```python
from build123d import *

# Parameters (mm, degrees)
RESSALTO_EXTRUS_O1_DEPTH = 52
ESBO_O2_R                = 2
CORTE_EXTRUS_O1_DEPTH    = 100
ESBO_O3_W                = 41
ESBO_O3_H                = 32.35
CORTE_EXTRUS_O2_DEPTH    = 8.5
ESBO_O8_W                = 65
ESBO_O8_H                = 5.3
CORTE_EXTRUS_O6_DEPTH    = 39
ESBO_O9_W                = 0.75
ESBO_O9_H                = 56.4
CORTE_EXTRUS_O7_DEPTH    = 45
FILETE6_R                = 8


with BuildPart() as part:
    # Esboço1 → Ressalto-extrusão1 (new body)
    with BuildSketch(Plane(origin=(0, 0, 0), x_dir=(1, 0, 0), z_dir=(0, 1, 0))):
        Polygon((-32.5, -28.2), (-20.5, -28.2), (-20.5, 28.2), (-32.5, 28.2), (-32.5, 33.5), (32.5, 33.5), (32.5, 28.2), (20.5, 28.2), (20.5, -28.2), (32.5, -28.2), (32.5, -33.5), (-32.5, -33.5), align=None)
    extrude(amount=RESSALTO_EXTRUS_O1_DEPTH)

    # Esboço2 → Corte-extrusão1 (cut)
    with BuildSketch(Plane.XY.offset(33.5)):
        with Locations((27.8, 5.4)):
            Circle(ESBO_O2_R)
        with Locations((-27.8, 5.4)):
            Circle(ESBO_O2_R)
    extrude(amount=-CORTE_EXTRUS_O1_DEPTH, mode=Mode.SUBTRACT)

    # Esboço3 → Corte-extrusão2 (cut)
    with BuildSketch(Plane(origin=(0, 52, 0), x_dir=(1, 0, 0), z_dir=(0, 1, 0))):
        with Locations((0, -12.025)):
            Rectangle(ESBO_O3_W, ESBO_O3_H)
    extrude(amount=-CORTE_EXTRUS_O2_DEPTH, mode=Mode.SUBTRACT)

    # Esboço8 → Corte-extrusão6 (cut)
    with BuildSketch(Plane(origin=(0, 52, 0), x_dir=(1, 0, 0), z_dir=(0, 1, 0))):
        with Locations((0, -30.85)):
            Rectangle(ESBO_O8_W, ESBO_O8_H)
    extrude(amount=-CORTE_EXTRUS_O6_DEPTH, mode=Mode.SUBTRACT)

    # Esboço9 → Corte-extrusão7 (cut)
    with BuildSketch(Plane(origin=(0, 52, 0), x_dir=(1, 0, 0), z_dir=(0, 1, 0))):
        with Locations((-20.125, 0)):
            Rectangle(ESBO_O9_W, ESBO_O9_H)
        with Locations((20.125, 0)):
            Rectangle(ESBO_O9_W, ESBO_O9_H)
    extrude(amount=-CORTE_EXTRUS_O7_DEPTH, mode=Mode.SUBTRACT)

    # Filete6
    filete6_edges = [part.edges().sort_by_distance(p)[0] for p in [
        (19.75, 43.5, 12.025),
        (-19.75, 43.5, 12.025),
    ]]
    fillet(filete6_edges, radius=FILETE6_R)


solid = part.part
```
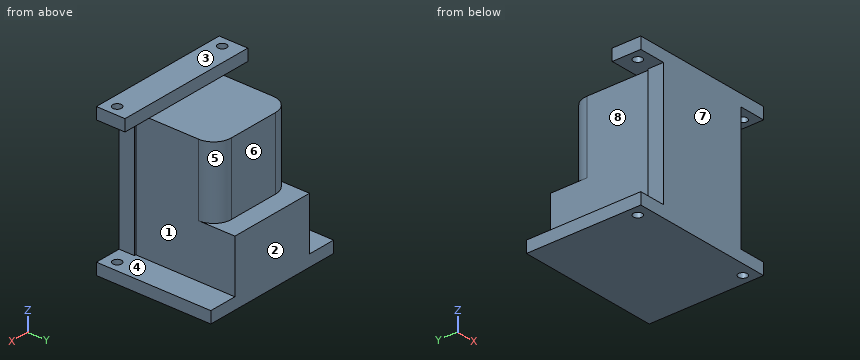
The listing builds one solid part. Answer for the finished solid, in the listing's coordinates (mm). Face numbers are marked on the shaded views. A direction names the side the tool comes from. Coordinates: 2 decimals unless noted, no trailing zeros. Loops run counter-clockwise (first coordinate to the right, second up) from the corner with the lowest first, then second, coordinate; pieces in that order, holes last. Notation, with made-up numbers: (9.25, 84.5) - (24.25, 84.5) arc R18 ccw to (24.25, 104.5) - close; hole circle Ø7 at (-18.5, 14.5). An arc over 180 degrees is marked (long way). Use a Markdown table: item, result. Add a question column.
1) The part is cut by section B-B, the plane y = 5.4. Give the vertices of the cut face in (x, z).
2) The part is cut by section C-C, the plane x = 27.8. Give the vertices of the cut face in (y, z).
3) The part is cut by section A-A, the plane z = -10. Give the vertices of the cut face in (x, y), and give its area (3 significant figures).
4) The mould has two halves that part along Z. Classify the marked faces 1, 2, 3 and 4: released by +Z, released by -Z, zero draft, split by the parting line, or undercut.
5) Find the intervals of material crossed by line 1 (Y direction, x = 27.8, z = -31.4); line 2 (X direction, y = 5, z = -29); line 3 (Z direction, x = 24, y = 10), in increasing order.
6) The part is cut by section D-D, the plane y = 22. Give the vertices of the cut face in (x, z).
7) Given pin 1 (3.5 mm diameter, centred on y = 3, z = 12.5, fed in from -X); pin 2 (5 mm diameter, centred on x = -6.5, y = 43, fed in from +Z); pin 3 (10 mm diameter, centred on y = 27.5, z = 22, fed in from +X), each flat-ended and moving along its own axis, determine where each tip first touches the part or whether it passes through.
8) For the marked faces 5, 6, 7 and 8, determine the directions among +Z, -Z, +X, -X, +Y, -Y from which every point of the face is accessible in a straight line to the end or side of a thin tool.
Here are the results:
| question | item | result |
|---|---|---|
| 1 | outline | (-32.5, -33.5) - (-29.8, -33.5) - (-29.8, -28.2) - (-32.5, -28.2) - close; (-32.5, 28.2) - (-29.8, 28.2) - (-29.8, 33.5) - (-32.5, 33.5) - close; (-25.8, -33.5) - (25.8, -33.5) - (25.8, -28.2) - (20.5, -28.2) - (20.5, 28.2) - (25.8, 28.2) - (25.8, 33.5) - (-25.8, 33.5) - (-25.8, 28.2) - (-20.5, 28.2) - (-20.5, -28.2) - (-25.8, -28.2) - close; (29.8, -33.5) - (32.5, -33.5) - (32.5, -28.2) - (29.8, -28.2) - close; (29.8, 28.2) - (32.5, 28.2) - (32.5, 33.5) - (29.8, 33.5) - close |
| 2 | outline | (0, -33.5) - (3.4, -33.5) - (3.4, -28.2) - (0, -28.2) - close; (0, 28.2) - (3.4, 28.2) - (3.4, 33.5) - (0, 33.5) - close; (7.4, -33.5) - (52, -33.5) - (52, -28.2) - (7.4, -28.2) - close; (7.4, 28.2) - (13, 28.2) - (13, 33.5) - (7.4, 33.5) - close |
| 3 | outline | (-20.5, 0) - (20.5, 0) - (20.5, 7) - (19.75, 7) - (19.75, 52) - (-19.75, 52) - (-19.75, 7) - (-20.5, 7) - close |
| 3 | area | 2,060 mm^2 |
| 4 | face 1 | undercut |
| 4 | face 2 | zero draft |
| 4 | face 3 | released by +Z |
| 4 | face 4 | undercut |
| 5 | line 1 | y = 0 to 3.4, 7.4 to 52 |
| 5 | line 2 | x = -32.5 to -29.76, -25.84 to 25.84, 29.76 to 32.5 |
| 5 | line 3 | z = -33.5 to -28.2, 28.2 to 33.5 |
| 6 | outline | (-32.5, -33.5) - (32.5, -33.5) - (32.5, -28.2) - (19.75, -28.2) - (19.75, 28.2) - (-19.75, 28.2) - (-19.75, -28.2) - (-32.5, -28.2) - close |
| 7 | pin 1 | stops at x = -20.5 |
| 7 | pin 2 | stops at z = 28.2 |
| 7 | pin 3 | stops at x = 19.75 |
| 8 | face 5 | +Z, +X, +Y |
| 8 | face 6 | +Z, +X, -X, +Y |
| 8 | face 7 | +Z, -Z, +X, -X, -Y |
| 8 | face 8 | -X, +Y |
